The listing builds one solid part. Answer for the finished solid, in the listing's coordinates (mm). A direction names the side the tool comes from. Coordinates: 2 decimals unless noted, no trailing zeros. Write each loop counter-clockwise with the first axis right and the second up, starting at its lowest first coordinate (ties: lowest second). Pieces come first, ordered by that corner, then holes. Notation, with made-up numbers: M 28.5,-38 L 50.5,-38 A12 ccw 50.5,-27 Z; hole C -20,-34.5 d7. An arc over 180 degrees is marked long. Answer as CSV lines item,"result".
```python
from build123d import *

# Parameters (mm, degrees)
SKETCH1_R           = 31
SKETCH1_R_2         = 30
BOSS_EXTRUDE1_DEPTH = 37
SKETCH2_R           = 31
BOSS_EXTRUDE2_DEPTH = 2
SKETCH5_R           = 30
SKETCH5_R_2         = 29.5
BOSS_EXTRUDE4_DEPTH = 2
SKETCH6_R           = 4
CUT_EXTRUDE1_DEPTH  = 2


with BuildPart() as part:
    # Sketch1 → Boss-Extrude1 (new body)
    with BuildSketch(Plane(origin=(0, 0, 0), x_dir=(1, 0, 0), z_dir=(0, 1, 0))):
        with Locations(Location((0, 0, 0), (0, 0, 270))):
            Circle(SKETCH1_R)
        with Locations(Location((0, 0, 0), (0, 0, 270))):
            Circle(SKETCH1_R_2, mode=Mode.SUBTRACT)
    extrude(amount=BOSS_EXTRUDE1_DEPTH)

    # Sketch2 → Boss-Extrude2 (add)
    with BuildSketch(Plane(origin=(0, 0, 0), x_dir=(1, 0, 0), z_dir=(0, 1, 0))):
        with Locations(Location((0, 0, 0), (0, 0, 270))):
            Circle(SKETCH2_R)
    extrude(amount=BOSS_EXTRUDE2_DEPTH)

    # Sketch5 → Boss-Extrude4 (add)
    with BuildSketch(Plane(origin=(0, 2, 0), x_dir=(1, 0, 0), z_dir=(0, 1, 0))):
        with Locations(Location((0, 0, 0), (0, 0, 270))):
            Circle(SKETCH5_R)
        with Locations(Location((0, 0, 0), (0, 0, 270))):
            Circle(SKETCH5_R_2, mode=Mode.SUBTRACT)
    extrude(amount=BOSS_EXTRUDE4_DEPTH)

    # Sketch6 → Cut-Extrude1 (cut)
    with BuildSketch(Plane(origin=(0, 2, 0), x_dir=(1, 0, 0), z_dir=(0, 1, 0))):
        with Locations(Location((0, 0, 0), (0, 0, 270))):
            Circle(SKETCH6_R)
    extrude(amount=-CUT_EXTRUDE1_DEPTH, mode=Mode.SUBTRACT)


solid = part.part
```
Q1. Find section B-B (z = 0). Give the vertices of the cut face in (x, y), and give its area (3 significant figures).
Output:
outline,"M -31,0 L -4,0 L -4,2 L -29.5,2 L -29.5,4 L -30,4 L -30,37 L -31,37 Z; M 4,0 L 31,0 L 31,37 L 30,37 L 30,4 L 29.5,4 L 29.5,2 L 4,2 Z"
area,"180 mm2"
Q2. Straight lines are drawn through the part: line 1 (X direction, y = 12, z = 0); line 2 (X direction, y = 3.3, z = 0); line 3 (Y direction, x = 11.5, z = 6). For each, find the intervals that lie inside material, in ascending order.
Output:
line 1,"-31 to -30, 30 to 31"
line 2,"-31 to -29.5, 29.5 to 31"
line 3,"0 to 2"
Q3. For faces 1 (the cylindrical face through (8.86, 2.99, 28.14)), 2 (the cylindrical face through (-3.905, 1.014, -0.867)), determine the directions among +Z, -Z, +X, -X, +Y, -Y from which every point of the face is accessible in a straight line to the end or side of a thin tool.
Output:
face 1,"+Y"
face 2,"+Y, -Y"
Q4. Find section C-C (y = 9.5). Give the vertices of the cut face in (x, z).
Output:
outline,"C 0,0 d62; hole C 0,0 d60"
Q5. Find section D-D (z = 17). Give the vertices of the cut face in (x, y), and give its area (3 significant figures).
Output:
outline,"M -25.92,0 L 25.92,0 L 25.92,37 L 24.72,37 L 24.72,4 L 24.11,4 L 24.11,2 L -24.11,2 L -24.11,4 L -24.72,4 L -24.72,37 L -25.92,37 Z"
area,"190 mm2"
Q6. The mould has two halves that part along X. Classify faces 3 (the flat face through (-20, 4, 22)), 4 (the cylindrical face through (30.736, 18.241, -4.036)), 5 (the flat face through (-6, 0, 0)): pulls with the +X half, pulls with the -X half, needs draft (parallel to the pull), parting line crosses it, or undercut.
Output:
face 3,"undercut"
face 4,"parting line crosses it"
face 5,"needs draft"
Q7. Find section A-A (x = 0). Give the vertices of the cut face in (y, z).
Output:
outline,"M 0,-31 L 37,-31 L 37,-30 L 4,-30 L 4,-29.5 L 2,-29.5 L 2,-4 L 0,-4 Z; M 0,4 L 2,4 L 2,29.5 L 4,29.5 L 4,30 L 37,30 L 37,31 L 0,31 Z"
Q8. Flat-ended cylindrical pins translate along their axes: pin 1 Ø1 at (x, y) = (18, 13.5) entering from -Z; pin 2 Ø4 at (x, z) = (-22.5, 13.5) entering from +Y; pin 3 Ø1.5 at (x, y) = (14, 14.5) entering from +Z. Find the tip coordinate at first contact, or state that the pin passes through.
Output:
pin 1,"z = -25.59"
pin 2,"y = 2"
pin 3,"z = 28.03"
